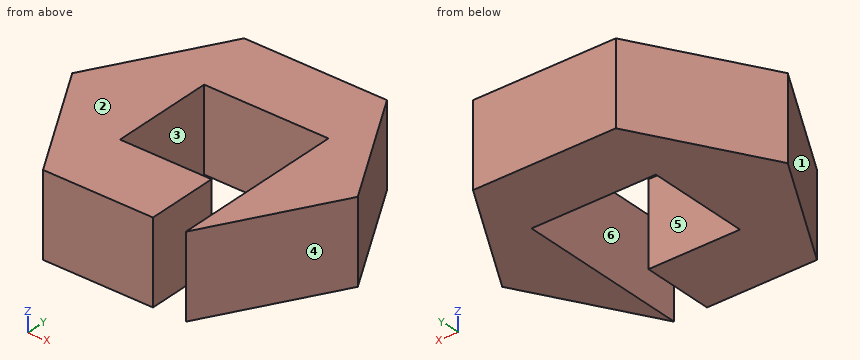
```python
from build123d import *

# Parameters (mm, degrees)
BOSS_EXTRUDE1_DEPTH = 10
SKETCH2_W           = 12.8478013
SKETCH2_H           = 12.538959922
CUT_EXTRUDE1_DEPTH  = 11
CUT_EXTRUDE3_START  = -21.26948
SKETCH3_W           = 3.975573171
SKETCH3_H           = 10
CUT_EXTRUDE3_DEPTH  = 21.26948


with BuildPart() as part:
    # Sketch1 → Boss-Extrude1 (new body)
    with BuildSketch(Plane.XY):
        Polygon((17.320508076, 0), (8.660254038, 15), (-8.660254038, 15), (-17.320508076, 0), (-8.660254038, -15), (8.660254038, -15), align=None)
    extrude(amount=BOSS_EXTRUDE1_DEPTH)

    # Sketch2 → Cut-Extrude1 (cut, through all)
    with BuildSketch(Plane.XY.offset(10)):
        Rectangle(SKETCH2_W, SKETCH2_H)
    extrude(amount=-CUT_EXTRUDE1_DEPTH, mode=Mode.SUBTRACT)

    # Sketch3 → Cut-Extrude3 (cut)
    with BuildSketch(Plane.XZ.offset(15).offset(CUT_EXTRUDE3_START)):
        with Locations((6.672467452, 5)):
            Rectangle(SKETCH3_W, SKETCH3_H)
    extrude(amount=CUT_EXTRUDE3_DEPTH, mode=Mode.SUBTRACT)


solid = part.part
```
For this review, take the finished solid that the model builds, in its own axes (mm). Face numbers are marked on the shaded views. A direction names the side the tool comes from. Coordinates: 2 decimals unless noted, no trailing zeros. Write each loop counter-clockwise with the first axis right and the second up, starting at its lowest first coordinate (ties: lowest second). Pieces come first, ordered by that corner, then holes. Notation, with made-up numbers: (-10, 72.25) - (36, 72.25) arc R16 ccw to (36, 80.25) - close; hole circle Ø3 at (-27, -22.75). An arc over 180 degrees is marked (long way). Put each result on its own line as item: value.
1. Add section D-D, the plane y = 7.5. Give the boundary of the cut face in (x, z).
Values found:
outline: (-12.99, 0) - (12.99, 0) - (12.99, 10) - (-12.99, 10) - close
2. Add section A-A, the plane y = -8.5. Give the boundary of the cut face in (x, z), then the cut area to 3 significant figures.
Values found:
outline: (-12.41, 0) - (4.68, 0) - (4.68, 10) - (-12.41, 10) - close; (8.66, 0) - (12.41, 0) - (12.41, 10) - (8.66, 10) - close
area: 209 mm²
3. Add section C-C, the plane z = 1. Give the boundary of the cut face in (x, y).
Values found:
outline: (-17.32, 0) - (-8.66, -15) - (4.68, -15) - (4.68, -6.27) - (-6.42, -6.27) - (-6.42, 6.27) - (8.66, 6.27) - (8.66, -15) - (17.32, 0) - (8.66, 15) - (-8.66, 15) - close
4. Machinability: for the marked faces 4, 5 and 6, which of the approach directions +Z, -Z, +X, -X, +Y, -Y give a long, thin tool a straight path to every point of the face, cutting with its end or side? Answer none if there is none.
Values found:
face 4: +Z, -Z, +X, -Y
face 5: +Z, -Z
face 6: +Z, -Z, -Y
5. Wall thickness on probe 1 along Y at (x, z) = (4, 5); probe 2 along X at (y, z) = (-13.25, 4.75); probe 3 along Y at (x, z) = (7, 2.75): over which ranges is each line inside the solid? List them lowest first.
Values found:
probe 1: -15 to -6.27, 6.27 to 15
probe 2: -9.67 to 4.68, 8.66 to 9.67
probe 3: 6.27 to 15
6. Add section B-B, the plane x = 3. Give the boundary of the cut face in (y, z), then the cut area to 3 significant figures.
Values found:
outline: (-15, 0) - (-6.27, 0) - (-6.27, 10) - (-15, 10) - close; (6.27, 0) - (15, 0) - (15, 10) - (6.27, 10) - close
area: 175 mm²
7. For pin 1 (2.5 mm diameter, centred on y = -12.5, z = 5.5, fed in from +X); pin 2 (2 mm diameter, centred on x = -10, z = 5.5, fed in from +Y); pin 3 (1 mm diameter, centred on y = -9, z = 7, fed in from +X), all flat-tipped, find the tip position at first contact; note any pin that passes through.
Values found:
pin 1: x = 10.83
pin 2: y = 14.41
pin 3: x = 12.41
8. Mouldability with a two-part tool opening along Y and no side actions: class the marked faces 1, 2 and 3 as released by +Y, released by -Y, zero draft, split by the parting line, or undercut.
Values found:
face 1: released by -Y
face 2: zero draft
face 3: undercut
